```python
from build123d import *

# Parameters (mm, degrees)
SKETCH1_W           = 15
SKETCH1_H           = 20
SKETCH1_R           = 2.5
BOSS_EXTRUDE1_DEPTH = 1
SKETCH2_W           = 15
SKETCH2_H           = 20
SKETCH2_R           = 2.5
BOSS_EXTRUDE2_DEPTH = 1


with BuildPart() as part:
    # Sketch1 → Boss-Extrude1 (new body)
    with BuildSketch(Plane(origin=(0, 0, 0), x_dir=(1, 0, 0), z_dir=(0, 1, 0))):
        Rectangle(SKETCH1_W, SKETCH1_H)
        with Locations(Location((0, 0, 0), (0, 0, 270))):
            Circle(SKETCH1_R, mode=Mode.SUBTRACT)
    extrude(amount=BOSS_EXTRUDE1_DEPTH)

    # Sketch2 → Boss-Extrude2 (add)
    with BuildSketch(Plane.XY.offset(10)):
        with Locations((0, 10)):
            Rectangle(SKETCH2_W, SKETCH2_H)
        with Locations((0, 10)):
            Circle(SKETCH2_R, mode=Mode.SUBTRACT)
    extrude(amount=BOSS_EXTRUDE2_DEPTH)


solid = part.part
```
Can you work these out from the model? Positions are in its coordinate system, mm. A direction names the side the tool comes from. Coordinates: 2 decimals unless noted, no trailing zeros. Order: outer loops, then holes, each group sorted by start corner. A loop starts at its lowest first (then second) coordinate and runs counter-clockwise, first axis right, second up. Notation, with made-up numbers: (48, -24.5) - (104, -24.5) arc R10 ccw to (104, -14.5) - close; hole circle Ø11 at (74, -13). An arc over 180 degrees is marked (long way). Answer in a Markdown table with one row per item.
1. Suppose I cut it at A-A (y = 10). Please give me the cut outline in (x, z), and give its area (3 significant figures).
Reply:
| item | result |
|---|---|
| outline | (-7.5, 10) - (-2.5, 10) - (-2.5, 11) - (-7.5, 11) - close; (2.5, 10) - (7.5, 10) - (7.5, 11) - (2.5, 11) - close |
| area | 10.0 mm^2 |
2. Suppose I cut it at C-C (x = 0). Please give me the cut outline in (y, z), and give its area (3 significant figures).
Reply:
| item | result |
|---|---|
| outline | (0, -10) - (1, -10) - (1, -2.5) - (0, -2.5) - close; (0, 2.5) - (1, 2.5) - (1, 10) - (7.5, 10) - (7.5, 11) - (0, 11) - close; (12.5, 10) - (20, 10) - (20, 11) - (12.5, 11) - close |
| area | 30.0 mm^2 |
3. If we mould it in two halves opening along X, with no side actions, what happens to faces 1 (the cylindrical face through (-0.54, 7.56, 10.49)), 2 (the flat face through (0, 0, 3)), 3 (the cylindrical face through (-2.44, 0.49, -0.54)), 4 (the flat face through (-7.5, 0.3, 5.1))? For each: pulls with the +X half, pulls with the -X half, needs draft (parallel to the pull), parting line crosses it, or undercut.
Reply:
| item | result |
|---|---|
| face 1 | undercut |
| face 2 | needs draft |
| face 3 | undercut |
| face 4 | pulls with the -X half |
4. Suppose I cut it at B-B (z = 0). Please give me the cut outline in (x, y), and give its area (3 significant figures).
Reply:
| item | result |
|---|---|
| outline | (-7.5, 0) - (-2.5, 0) - (-2.5, 1) - (-7.5, 1) - close; (2.5, 0) - (7.5, 0) - (7.5, 1) - (2.5, 1) - close |
| area | 10.0 mm^2 |
5. If I drill on line 1 along Y through (x, z) = (0, 10.5); line 2 along X through (y, z) = (0.3, 0); line 3 along Y through (x, z) = (-6, 8), over which ranges is the centre line in solid material (lowest first)?
Reply:
| item | result |
|---|---|
| line 1 | y = 0 to 7.5, 12.5 to 20 |
| line 2 | x = -7.5 to -2.5, 2.5 to 7.5 |
| line 3 | y = 0 to 1 |
6. For pin 1 (2 mm diameter, centred on x = -0.5, y = 17, fed in from -Z); pin 2 (1.5 mm diameter, centred on x = 1.5, z = 5, fed in from +Y), each with a flat end and sliding along its axis, tell me the tip position at first contact or that it passes through.
Reply:
| item | result |
|---|---|
| pin 1 | stops at z = 10 |
| pin 2 | stops at y = 1 |
7. Suppose I cut it at D-D (z = -8). Please give me the cut outline in (x, y), and give its area (3 significant figures).
Reply:
| item | result |
|---|---|
| outline | (-7.5, 0) - (7.5, 0) - (7.5, 1) - (-7.5, 1) - close |
| area | 15.0 mm^2 |
8. For faces 5 (the flat face through (-2, 12, 11)), 6 (the flat face through (0, 13, 10)), which set-ups out of +Z, -Z, +X, -X, +Y, -Y let a thin tool reach every point of the face, with its end or its side?
Reply:
| item | result |
|---|---|
| face 5 | +Z, +X, -X, +Y, -Y |
| face 6 | -Z, +X, -X, +Y |
